```python
from build123d import *

# Parameters (mm, degrees)
F0_R     = 2.54
F1_DEPTH = 5.08


with BuildPart() as f1:
    # F0 (on Top) → F1 (new body)
    with BuildSketch(Plane.XY):
        with BuildLine():
            ThreePointArc((-33.02, 38.1), (-34.5078975516, 41.6921024484), (-38.1, 43.18))
            ThreePointArc((-38.1, 43.18), (-41.6921024484, 41.6921024484), (-43.18, 38.1))
            ThreePointArc((-43.18, 38.1), (-38.1, 33.02), (-33.02, 38.1))
        make_face()
        with BuildLine():
            ThreePointArc((-43.18, -38.1), (-41.6921024484, -41.6921024484), (-38.1, -43.18))
            ThreePointArc((-38.1, -43.18), (-34.5078975516, -41.6921024484), (-33.02, -38.1))
            ThreePointArc((-33.02, -38.1), (-38.1, -33.02), (-43.18, -38.1))
        make_face()
        with BuildLine():
            Line((0, 43.18), (0, 38.1))
            Line((0, 38.1), (33.02, 38.1))
            ThreePointArc((33.02, 38.1), (34.5078975516, 41.6921024484), (38.1, 43.18))
            Line((38.1, 43.18), (0, 43.18))
        make_face()
        with BuildLine():
            Line((38.1, 33.02), (38.1, 0))
            Line((38.1, 0), (43.18, 0))
            Line((43.18, 0), (43.18, 38.1))
            ThreePointArc((43.18, 38.1), (41.6921024484, 34.5078975516), (38.1, 33.02))
        make_face()
        with BuildLine():
            Line((38.1, 38.1), (38.1, 33.02))
            ThreePointArc((38.1, 33.02), (41.6921024484, 34.5078975516), (43.18, 38.1))
            ThreePointArc((43.18, 38.1), (42.795516496, 40.0386915268), (41.7002658126, 41.68392049))
            Line((41.7002658126, 41.68392049), (38.1, 38.1))
        make_face()
        with BuildLine():
            ThreePointArc((38.1, 43.18), (34.5078975516, 41.6921024484), (33.02, 38.1))
            Line((33.02, 38.1), (38.1, 38.1))
            Line((38.1, 38.1), (41.7002658126, 41.68392049))
            ThreePointArc((41.7002658126, 41.68392049), (40.0493696303, 42.7910934807), (38.1, 43.18))
        make_face()
        with BuildLine():
            Line((38.1, 38.1), (33.02, 38.1))
            ThreePointArc((33.02, 38.1), (33.4066919748, 36.1559681636), (34.5078975516, 34.5078975516))
            Line((34.5078975516, 34.5078975516), (38.1, 38.1))
        make_face()
        with BuildLine():
            ThreePointArc((34.5078975516, 34.5078975516), (36.1559681636, 33.4066919748), (38.1, 33.02))
            Line((38.1, 33.02), (38.1, 38.1))
            Line((38.1, 38.1), (34.5078975516, 34.5078975516))
        make_face()
        with BuildLine():
            ThreePointArc((38.1, -43.18), (41.6921024484, -41.6921024484), (43.18, -38.1))
            ThreePointArc((43.18, -38.1), (34.5078975516, -34.5078975516), (38.1, -43.18))
        make_face()
        with BuildLine():
            Line((38.1, 0), (20.32, 0))
            ThreePointArc((20.32, 0), (8.2713308178, -18.5603740938), (-13.5862486715, -15.1101372275))
            ThreePointArc((-13.5862486715, -15.1101372275), (-18.9728804938, 7.2754522724), (0, 20.32))
            Line((0, 20.32), (0, 38.1))
            Line((0, 38.1), (0, 43.18))
            Line((0, 43.18), (-38.1, 43.18))
            ThreePointArc((-38.1, 43.18), (-34.5078975516, 41.6921024484), (-33.02, 38.1))
            ThreePointArc((-33.02, 38.1), (-38.1, 33.02), (-43.18, 38.1))
            Line((-43.18, 38.1), (-43.18, 0))
            Line((-43.18, 0), (-43.18, -38.1))
            ThreePointArc((-43.18, -38.1), (-38.1, -33.02), (-33.02, -38.1))
            ThreePointArc((-33.02, -38.1), (-34.5078975516, -41.6921024484), (-38.1, -43.18))
            Line((-38.1, -43.18), (0, -43.18))
            Line((0, -43.18), (38.1, -43.18))
            ThreePointArc((38.1, -43.18), (34.5078975516, -34.5078975516), (43.18, -38.1))
            Line((43.18, -38.1), (43.18, 0))
            Line((43.18, 0), (38.1, 0))
        make_face()
        with Locations((-28.7368195874, -28.7368195874)):
            Circle(F0_R, mode=Mode.SUBTRACT)
        with Locations((28.7368195874, -28.7368195874)):
            Circle(F0_R, mode=Mode.SUBTRACT)
        with Locations((-28.7368195874, 28.7368195874)):
            Circle(F0_R, mode=Mode.SUBTRACT)
        with BuildLine():
            ThreePointArc((14.3684097937, 14.3684097937), (18.7732321006, 7.7761273457), (20.32, 0))
            Line((20.32, 0), (38.1, 0))
            Line((38.1, 0), (38.1, 33.02))
            ThreePointArc((38.1, 33.02), (36.1559681636, 33.4066919748), (34.5078975516, 34.5078975516))
            Line((34.5078975516, 34.5078975516), (30.5328708116, 30.5328708116))
            ThreePointArc((30.5328708116, 30.5328708116), (31.0834736, 29.7088355056), (31.2768195874, 28.7368195874))
            ThreePointArc((31.2768195874, 28.7368195874), (29.7088355056, 26.3901655748), (26.9407683632, 26.9407683632))
            Line((26.9407683632, 26.9407683632), (14.3684097937, 14.3684097937))
        make_face()
        with BuildLine():
            Line((0, 38.1), (0, 20.32))
            ThreePointArc((0, 20.32), (7.7761273457, 18.7732321006), (14.3684097937, 14.3684097937))
            Line((14.3684097937, 14.3684097937), (26.9407683632, 26.9407683632))
            ThreePointArc((26.9407683632, 26.9407683632), (26.2202806744, 28.3923897696), (26.5242217024, 29.9842211264))
            ThreePointArc((26.5242217024, 29.9842211264), (28.3923897696, 31.2533585004), (30.5328708116, 30.5328708116))
            Line((30.5328708116, 30.5328708116), (34.5078975516, 34.5078975516))
            ThreePointArc((34.5078975516, 34.5078975516), (33.4066919748, 36.1559681636), (33.02, 38.1))
            Line((33.02, 38.1), (0, 38.1))
        make_face()
    extrude(amount=F1_DEPTH)


solid = f1.part
```
The model under review builds one solid part; all positions refer to its coordinate system, in mm. Coordinates: 2 decimals unless noted, no trailing zeros. Write each loop counter-clockwise with the first axis right and the second up, starting at its lowest first coordinate (ties: lowest second). Pieces come first, ordered by that corner, then holes.
1) To check wall thickness, follow probe 1 along X at (y, z) = (29, 4.3); probe 2 along Y at (x, z) = (-27, 4.1); probe 3 along X at (y, z) = (-29.5, 2.85). State the ranges of each line that lie inside material, in increasing order.
2) We need section A-A on x = 0. State the section outline as (y, z) points, then the cut area to 3 significant figures.
3) We need section D-D on x = -29. State the section outline as (y, z) points.
4) Clearance check with a flat-ended pin moving along its axis: pin 1 Ø6.5 at (x, y) = (-28.74, -28.74) entering from +Z. State where the tip first meets the part, or that it passes through.
5) We need section C-C on y = -11.5. State the section outline as (x, z) points, then the cut area to 3 significant figures.
6) The part is to be moulded in two halves that separate along Y. For faces 1 (the face through (1, 43.18, 3)), 2 (the face through (-20, 10, 0)), 3 (the face through (-1, -43.18, 3)), 4 (the face through (-30.752, -30.282, 2.504)), say which applies: pulls with the +Y half, pulls with the -Y half, needs draft (parallel to the pull), parting line crosses it, or undercut.
7) We need section B-B on z = 2.55. State the section outline as (x, y) points, then the cut area to 3 significant figures.
Answer list:
1. probe 1: x = -43.18 to -31.26, -26.21 to 26.21, 31.26 to 43.18
1. probe 2: y = -43.18 to -30.59, -26.88 to 26.88, 30.59 to 43.18
1. probe 3: x = -43.18 to -31.16, -26.31 to 26.31, 31.16 to 43.18
2. outline: (-43.18, 0) - (-20.32, 0) - (-20.32, 5.08) - (-43.18, 5.08) - close; (20.32, 0) - (43.18, 0) - (43.18, 5.08) - (20.32, 5.08) - close
2. area: 232 mm2
3. outline: (-43.18, 0) - (-31.26, 0) - (-31.26, 5.08) - (-43.18, 5.08) - close; (-26.21, 0) - (26.21, 0) - (26.21, 5.08) - (-26.21, 5.08) - close; (31.26, 0) - (43.18, 0) - (43.18, 5.08) - (31.26, 5.08) - close
4. pin 1: stops at z = 5.08
5. outline: (-43.18, 0) - (-16.75, 0) - (-16.75, 5.08) - (-43.18, 5.08) - close; (16.75, 0) - (43.18, 0) - (43.18, 5.08) - (16.75, 5.08) - close
5. area: 269 mm2
6. face 1: pulls with the +Y half
6. face 2: needs draft
6. face 3: pulls with the -Y half
6. face 4: undercut
7. outline: (-43.18, -38.1) arc R5.08 ccw to (-38.1, -43.18) - (38.1, -43.18) arc R5.08 ccw to (43.18, -38.1) - (43.18, 38.1) arc R5.08 ccw to (38.1, 43.18) - (-38.1, 43.18) arc R5.08 ccw to (-43.18, 38.1) - close; hole circle Ø5.08 at (-28.74, -28.74); hole circle Ø5.08 at (-28.74, 28.74); hole circle Ø40.64 at (0, 0); hole circle Ø5.08 at (28.74, -28.74); hole circle Ø5.08 at (28.74, 28.74)
7. area: 6,060 mm2
